Could you check a few things on this model? Use its own coordinates, in mm. Face numbers are marked on the shaded views. A direction names the side the tool comes from. Round coordinates to 2 decimals unless told otherwise and drop trailing zeros. Order: outer loops, then holes, each group sorted by start corner. A loop starts at its lowest first (then second) coordinate and runs counter-clockwise, first axis right, second up. Notation, with made-up numbers: (-34, -15.5) - (17, -15.5) arc R37 ccw to (17, 22.5) - close; hole circle Ø6 at (80.5, 3.5). An arc over 180 degrees is marked (long way). Use one line per item in the form item = value.
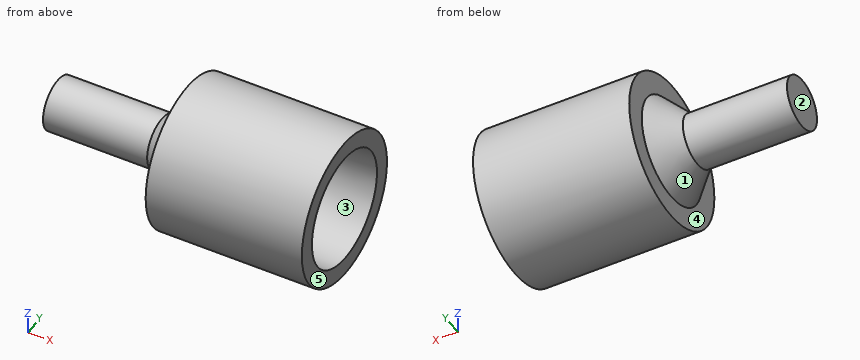
from build123d import *

# Parameters (mm, degrees)
CHAMFER_1_SIZE = 3


with BuildPart() as part:
    # 草图1 → 旋转1 (revolve)
    with BuildSketch(Plane(origin=(0, 0, 0), x_dir=(1, 0, 0), z_dir=(0, 1, 0))):
        Polygon((15, 8.5), (-3, 8.5), (-3, 3), (-18, 3), (-18, 0), (0, 0), (0, 5.75), (15, 6.5), align=None)
    revolve(axis=Axis((-18, 0, 0), (1, 0, 0)))

    # 倒角1
    chamfer_1_edges = [part.edges().sort_by_distance(p)[0] for p in [
        (-3, 0, 3),
    ]]
    chamfer(chamfer_1_edges, length=CHAMFER_1_SIZE)


solid = part.part
Item 1: Imagine slicing it at C-C on x = -12. Please give me the cut outline in (y, z).
Found:
outline = circle Ø6 at (0, 0)
Item 2: Will these pins go through, and if not, where does the flat tip stop? P1, Ø1, axis at y = 0, z = -4, coming from the +X side; P2, Ø1.5, axis at x = -1, z = -4.5, coming from the +Y side; P3, Ø3, axis at x = 0, z = -4, coming from the +Y side.
Found:
P1 = 0
P2 = 7.63
P3 = 8.12
Item 3: For the marked faces 4 and 5, which set-ups out of +Z, -Z, +X, -X, +Y, -Y let a thin tool reach every point of the face, with its end or its side?
Found:
face_4 = -X
face_5 = +Z, -Z, +X, +Y, -Y
Item 4: I need wall thicknesses on L1, parallel to Y at x = 7.5, z = 3.75; L2, parallel to Z at x = 7.5, y = -1; L3, parallel to X at y = -6.5, z = -2.5. Which ranges of each line are inside material? Lowest first, please.
Found:
L1 = -7.63 to -4.84, 4.84 to 7.63
L2 = -8.44 to -6.04, 6.04 to 8.44
L3 = -3 to 15
Item 5: If we mould it in two halves opening along Z, with no side actions, what happens to the marked faces 1, 2 and 3? For each: released by +Z, released by -Z, zero draft, split by the parting line, or undercut.
Found:
face_1 = split by the parting line
face_2 = zero draft
face_3 = undercut
Item 6: Imagine slicing it at A-A on y = 0. Please give me the cut outline in (x, z), plus the area to 3 significant figures.
Found:
outline = (-18, -3) - (-6, -3) - (-3, -6) - (-3, -8.5) - (15, -8.5) - (15, -6.5) - (0, -5.75) - (0, 5.75) - (15, 6.5) - (15, 8.5) - (-3, 8.5) - (-3, 6) - (-6, 3) - (-18, 3) - close
area = 221 mm2
Item 7: Imagine slicing it at D-D on x = 4. Please give me the cut outline in (y, z).
Found:
outline = circle Ø17 at (0, 0); hole circle Ø11.9 at (0, 0)
